CAD build for the part. Positions are in the model's coordinates, mm. A direction names the side the tool comes from. Coordinates: 2 decimals unless noted, no trailing zeros. Write each loop counter-clockwise with the first axis right and the second up, starting at its lowest first coordinate (ties: lowest second). Pieces come first, ordered by that corner, then holes. Notation, with made-up numbers: M 41,4.25 L 79,4.25 A22 cw 79,34.25 Z; hole C 46.25,-24.75 d11. An arc over 180 degrees is marked long. Answer as CSV lines item,"result". Start each with the question number.
```python
from build123d import *

# Parameters (mm, degrees)
SKETCH_1_W      = 230
SKETCH_1_H      = 80
SKETCH_1_R      = 3.5
SKETCH_1_R_2    = 4
SKETCH_1_R_3    = 6
SKETCH_1_W_2    = 52
SKETCH_1_H_2    = 41
SKETCH_1_W_3    = 26
SKETCH_1_H_3    = 12
SKETCH_1_W_4    = 24
SKETCH_1_H_4    = 10
EXTRUDE_1_DEPTH = 2
SKETCH_3_W      = 66.2
SKETCH_3_H      = 46.5
SKETCH_3_W_2    = 63.2
SKETCH_3_H_2    = 43.5
SKETCH_3_W_3    = 31
SKETCH_3_H_3    = 27.5
SKETCH_3_W_4    = 28
SKETCH_3_H_4    = 24.5
EXTRUDE_2_DEPTH = 6


with BuildPart() as part:
    # 草图1 → 凸台-拉伸1 (new body)
    with BuildSketch(Plane(origin=(0, 0, 0), x_dir=(1, 0, 0), z_dir=(0, 1, 0))):
        with Locations((23.568232821, 7.271766922)):
            Rectangle(SKETCH_1_W, SKETCH_1_H)
        with Locations(Location((-68.131767179, -14.128233078, 0), (0, 0, 270))):
            Circle(SKETCH_1_R, mode=Mode.SUBTRACT)
        with Locations(Location((-7.811767179, 29.771766922, 0), (0, 0, 270))):
            Circle(SKETCH_1_R, mode=Mode.SUBTRACT)
        with Locations(Location((-7.811767179, 19.071766922, 0), (0, 0, 270))):
            Circle(SKETCH_1_R, mode=Mode.SUBTRACT)
        with Locations(Location((-7.811767179, 8.371766922, 0), (0, 0, 270))):
            Circle(SKETCH_1_R, mode=Mode.SUBTRACT)
        with Locations(Location((-7.811767179, -2.328233078, 0), (0, 0, 270))):
            Circle(SKETCH_1_R, mode=Mode.SUBTRACT)
        with Locations(Location((16.688232821, 30.896203348, 0), (0, 0, 270))):
            Circle(SKETCH_1_R, mode=Mode.SUBTRACT)
        with Locations(Location((16.688232821, 18.896203348, 0), (0, 0, 270))):
            Circle(SKETCH_1_R, mode=Mode.SUBTRACT)
        with Locations(Location((16.688232821, 6.896203348, 0), (0, 0, 270))):
            Circle(SKETCH_1_R, mode=Mode.SUBTRACT)
        with Locations(Location((4.688232821, 18.896203348, 0), (0, 0, 270))):
            Circle(SKETCH_1_R, mode=Mode.SUBTRACT)
        with Locations(Location((28.688232821, 18.896203348, 0), (0, 0, 270))):
            Circle(SKETCH_1_R, mode=Mode.SUBTRACT)
        with Locations(Location((49.688232821, 18.896203348, 0), (0, 0, 270))):
            Circle(SKETCH_1_R_2, mode=Mode.SUBTRACT)
        with Locations(Location((59.568232821, -13.103233078, 0), (0, 0, 270))):
            Circle(SKETCH_1_R_2, mode=Mode.SUBTRACT)
        with Locations(Location((39.568232821, -13.103233078, 0), (0, 0, 270))):
            Circle(SKETCH_1_R_2, mode=Mode.SUBTRACT)
        with Locations(Location((126.568232821, 27.271766922, 0), (0, 0, 270))):
            Circle(SKETCH_1_R, mode=Mode.SUBTRACT)
        with Locations(Location((108.568232821, 2.271766922, 0), (0, 0, 270))):
            Circle(SKETCH_1_R_3, mode=Mode.SUBTRACT)
        with Locations((-42.431767179, 13.771766922)):
            Rectangle(SKETCH_1_W_2, SKETCH_1_H_2, mode=Mode.SUBTRACT)
        with Locations((99.568232821, 27.271766922)):
            Rectangle(SKETCH_1_W_3, SKETCH_1_H_3, mode=Mode.SUBTRACT)
        with Locations((108.568232821, -13.103233078)):
            Rectangle(SKETCH_1_W_4, SKETCH_1_H_4, mode=Mode.SUBTRACT)
    extrude(amount=EXTRUDE_1_DEPTH)

    # 草图3 → 凸台-拉伸2 (add)
    # profile 1 of 2: a face of its own
    with BuildSketch(Plane.XZ):
        with Locations((-46.831767179, -13.521766922)):
            Rectangle(SKETCH_3_W, SKETCH_3_H)
        with Locations((-46.831767179, -13.521766922)):
            Rectangle(SKETCH_3_W_2, SKETCH_3_H_2, mode=Mode.SUBTRACT)
    # profile 2 of 2: a face of its own
    with BuildSketch(Plane.XZ):
        with Locations((99.568232821, -23.521766922)):
            Rectangle(SKETCH_3_W_3, SKETCH_3_H_3)
        with Locations((99.568232821, -23.521766922)):
            Rectangle(SKETCH_3_W_4, SKETCH_3_H_4, mode=Mode.SUBTRACT)
    extrude(amount=EXTRUDE_2_DEPTH)


solid = part.part
```
1) Band-saw the part on A-A, the plane y = -2. List the corners of the cut face in (x, z), plus the area to 3 significant figures.
2) Tool access for faces 4 (the flat face through (-47, -3, 9.728)), 5 (the flat face through (-13.732, -3, -14)), 6 (the cylindrical face through (31.639, 0.986, -17.015)), 7 (the flat face through (-79.932, -3, -14)), 8 (the flat face through (99, -3, -11.272)): list every direction of +Z, -Z, +X, -X, +Y, -Y with a clear straight run to the whole face (end or side of a thin tool).
3) Band-saw the part on D-D, the plane z = 26.5. List the corners of the cut face in (x, y), plus the area to 3 significant figures.
4) Band-saw the part on B-B, the plane x = -39. List the corners of the cut face in (y, z), plus the area to 3 significant figures.
5) Band-saw the part on C-C, the plane z = -18. State how many separate pieces and enclosed holes the cut face has, plus the area to 3 significant figures.
6) Probe L1, parallel to X at y = -3.5, z = -20; L2, parallel to Z at x = -16, y = -2.5; L3, parallel to Z at x = 105, y = -1.25. List the from-to ranges inside material, lowest first. Write a range as [from, to].
7) Pin check, flat tips, straight feed: P1, Ø1.5, axis at x = 58, z = -28, coming from the -Y side; P2, Ø1.8, axis at y = -3.5, z = -19.5, coming from the +X side; P3, Ø1.8, axis at y = -3.5, z = -22.5, coming from the -X side. Stop position of each tip, or through.
8) Two-plate mould, pull along X, no slides. Class faces 1 (the cylindrical face through (5.74, 0.99, -15.56)), 2 (the flat face through (-47, -3, -36.772)), 3 (the flat face through (115.068, -3, -24)): pulls with the +X half, pulls with the -X half, needs draft (parallel to the pull), parting line crosses it, or undercut.
Result sheet:
1,outline,"M -79.93,-36.77 L -13.73,-36.77 L -13.73,9.73 L -79.93,9.73 Z; M 84.07,-37.27 L 115.07,-37.27 L 115.07,-9.77 L 84.07,-9.77 Z; hole M -78.43,-35.27 L -15.23,-35.27 L -15.23,8.23 L -78.43,8.23 Z; hole M 85.57,-35.77 L 113.57,-35.77 L 113.57,-11.27 L 85.57,-11.27 Z"
1,area,"496 mm²"
2,face 4,"+Z, +X, -X, -Y"
2,face 5,"+Z, -Z, -Y"
2,face 6,"+Y, -Y"
2,face 7,"+Z, -Z, -X, -Y"
2,face 8,"-Y"
3,outline,"M -91.43,0 L 138.57,0 L 138.57,2 L -91.43,2 Z"
3,area,"460 mm²"
4,outline,"M -6,-36.77 L 0,-36.77 L 0,-47.27 L 2,-47.27 L 2,-34.27 L 0,-34.27 L 0,-35.27 L -6,-35.27 Z; M -6,8.23 L 0,8.23 L 0,6.73 L 2,6.73 L 2,32.73 L 0,32.73 L 0,9.73 L -6,9.73 Z"
4,area,"96.0 mm²"
5,separate pieces,"7"
5,enclosed holes,"0"
5,area,"322 mm²"
6,L1,"x = [-79.93, -78.43], [-15.23, -13.73], [84.07, 85.57], [113.57, 115.07]"
6,L2,"z = [-36.77, -35.27], [8.23, 9.73]"
6,L3,"z = [-37.27, -35.77], [-11.27, -9.77]"
7,P1,"stops at y = 0"
7,P2,"stops at x = 115.07"
7,P3,"stops at x = -79.93"
8,face 1,"undercut"
8,face 2,"needs draft"
8,face 3,"pulls with the +X half"
